Input: part model. Units: mm. Frame: model coordinates. A direction names the side the tool comes from. Give positions to 0.01 mm unless a question says otherwise; leave off trailing zeros. Order: outer loops, then holes, each group sorted by start corner. A loop starts at its lowest first (then second) coordinate and runs counter-clockwise, first axis right, second up. Notation, with made-up numbers: (23, 31) -> (43, 31) arc R19 cw to (43, 63) -> close; hole circle Ø11 at (-40, 8). An arc over 180 degrees is marked (long way). Use a Markdown table: item, result. Add a question column.
from build123d import *

# Parameters (mm, degrees)
F1_DEPTH = 19.05


with BuildPart() as f1:
    # F0 (on Front) → F1 (new body, symmetric)
    with BuildSketch(Plane.XZ):
        with BuildLine():
            Line((-63.5, -9.525), (63.5, -9.525))
            Line((63.5, -9.525), (63.5, 9.525))
            ThreePointArc((63.5, 9.525), (52.412089, 15.981047), (40.67581, 21.165838))
            Line((40.67581, 21.165838), (40.67581, 13.053685))
            ThreePointArc((40.67581, 13.053685), (37.875132, 5.161991), (35.90061, 13.299797))
            Line((35.90061, 13.299797), (35.90061, 22.846459))
            ThreePointArc((35.90061, 22.846459), (0, 28.575), (-35.90061, 22.846459))
            Line((-35.90061, 22.846459), (-35.90061, 13.299797))
            ThreePointArc((-35.90061, 13.299797), (-37.875132, 5.161991), (-40.67581, 13.053685))
            Line((-40.67581, 13.053685), (-40.67581, 21.165838))
            ThreePointArc((-40.67581, 21.165838), (-52.412089, 15.981047), (-63.5, 9.525))
            Line((-63.5, 9.525), (-63.5, -9.525))
        make_face()
    extrude(amount=F1_DEPTH, both=True)


solid = f1.part
Q1. Draft query along X for faces 3 (the cylindrical face through (52.57, -0.27, 15.9)), 4 (the cylindrical face through (0.511, -0.267, 28.574)), 5 (the cylindrical face through (-37.719, -0.267, 5.173)). Return one class per face: +X half, -X half, draft (parallel to the pull), parting line (faces both ways), or undercut.
Q2. Section query A-A (z = 11). Return loops of the section in (x, y), plus the area to 3 significant figures.
Q3. Section query C-C (x = 38.1). Return loops of the section in (y, z) (3 decimals), plus the area to 3 significant figures.
Q4. Ray query, line 1 (X direction, y = -11, z = 12.5); line 2 (X direction, y = 15, z = 16.5); line 3 (Z direction, x = -38.1, y = -1.5) (3 decimals). Return the intervals inside material, ascending.
Q5. First-contact query: pin 1 (3 mm diameter, centred on y = 11.5, z = 12.5, fed in from +X); pin 2 (2.5 mm diameter, centred on y = 8.5, z = 17, fed in from +X); pin 3 (7.5 mm diameter, centred on y = -5.5, z = 17, fed in from -X). Flat tips, straight axial feed; report the tip coordinate or a pass-through.
Q6. Section query B-B (y = -3.5). Return loops of the section in (x, z) (3 decimals).
Q7. Section query D-D (x = -13.5). Return loops of the section in (y, z) (3 decimals), plus the area to 3 significant figures.
Q8. Access query for faces 1 (the cylindrical face through (38.032, -0.267, 5.157)), 2 (the flat face through (40.676, 0, 17)). Directions: +Z, -Z, +X, -X, +Y, -Y. A direction counts if a zero-diameter tool reaches every point of the face in a straight line with its end or side. Return the directions, or none.
Solution:
| question | item | result |
|---|---|---|
| 1 | face 3 | +X half |
| 1 | face 4 | parting line |
| 1 | face 5 | undercut |
| 2 | outline | (-61.2, -19.05) -> (-42.21, -19.05) -> (-42.21, 19.05) -> (-61.2, 19.05) -> close; (-33.99, -19.05) -> (33.99, -19.05) -> (33.99, 19.05) -> (-33.99, 19.05) -> close; (42.21, -19.05) -> (61.2, -19.05) -> (61.2, 19.05) -> (42.21, 19.05) -> close |
| 2 | area | 4,040 mm² |
| 3 | outline | (-19.05, -9.525) -> (19.05, -9.525) -> (19.05, 5.156) -> (-19.05, 5.156) -> close |
| 3 | area | 559 mm² |
| 4 | line 1 | x = -58.74 to -41.3, -34.9 to 34.9, 41.3 to 58.74 |
| 4 | line 2 | x = -51.38 to -40.68, -35.9 to 35.9, 40.68 to 51.38 |
| 4 | line 3 | z = -9.525 to 5.156 |
| 5 | pin 1 | stops at x = 61.2 |
| 5 | pin 2 | stops at x = 52.86 |
| 5 | pin 3 | stops at x = -57.45 |
| 6 | outline | (-63.5, -9.525) -> (63.5, -9.525) -> (63.5, 9.525) arc R115.358 ccw to (40.676, 21.166) -> (40.676, 13.054) arc R4.369 cw (long way) to (35.901, 13.3) -> (35.901, 22.846) arc R115.358 ccw to (-35.901, 22.846) -> (-35.901, 13.3) arc R4.369 cw (long way) to (-40.676, 13.054) -> (-40.676, 21.166) arc R115.358 ccw to (-63.5, 9.525) -> close |
| 7 | outline | (-19.05, -9.525) -> (19.05, -9.525) -> (19.05, 27.782) -> (-19.05, 27.782) -> close |
| 7 | area | 1,420 mm² |
| 8 | face 1 | +Y, -Y |
| 8 | face 2 | +Z, +Y, -Y |
